from build123d import *

# Parameters (mm, degrees)
BOSS_EXTRUDE1_DEPTH  = 4.7625
M8_CLEARANCE_HOLE1_D = 9
CHAMFER1_SIZE        = 1


with BuildPart() as part:
    # Sketch1 → Boss-Extrude1 (new, symmetric)
    with BuildSketch(Plane.XY):
        Polygon((-17.5, -157.849025767), (5.340097423, -157.849025767), (157.849025767, -5.340097423), (157.849025767, 17.5), (39.267766953, 17.5), (-17.5, -39.267766953), align=None)
    extrude(amount=BOSS_EXTRUDE1_DEPTH, both=True)

    # M8 Clearance Hole1 (through all)
    with Locations(Plane.XY.offset(4.7625)):
        with Locations((0, -92.478445072), (144.956890143, 0), (92.478445072, 0), (0, -40), (0, -144.956890143), (40, 0)):
            Hole(M8_CLEARANCE_HOLE1_D / 2)

    # Chamfer1
    chamfer1_edges = [part.edges().sort_by_distance(p)[0] for p in [
        (157.849025767, 17.5, 0),
        (157.849025767, -5.340097423, 0),
        (5.340097423, -157.849025767, 0),
        (-17.5, -157.849025767, 0),
        (-17.5, -39.267766953, 0),
        (39.267766953, 17.5, 0),
    ]]
    chamfer(chamfer1_edges, length=CHAMFER1_SIZE)


solid = part.part
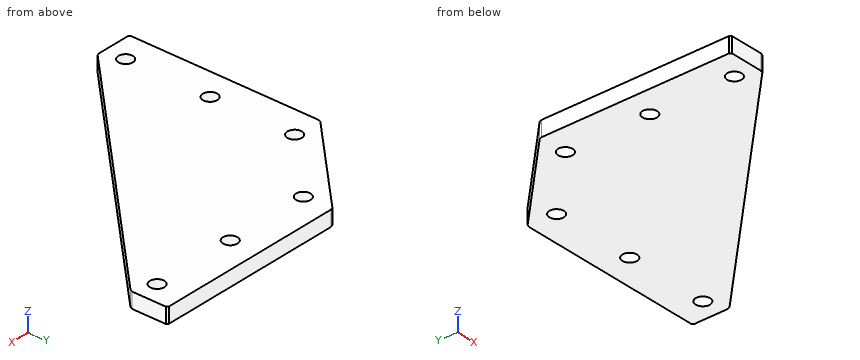
Geometry: final body of the model. Coordinates: model frame, mm. Give positions to 0.01 mm unless a question says otherwise; leave off trailing zeros. Write each loop counter-clockwise with the first axis right and the second up, starting at its lowest first coordinate (ties: lowest second). Pieces come first, ordered by that corner, then holes. Notation, with made-up numbers: (27.25, 56.5) - (65.25, 56.5) arc R13 cw to (65.25, 67.5) - close; hole circle Ø9 at (64.5, 24.5). An arc over 180 degrees is marked (long way). Return JSON: item names as keys, results as strings. Group by question number.
1) Section B-B on y = 0. Return the cut outline in (x, z).
2) First-contact query: P1, Ø7, axis at x = 0, y = -40, coming from the -Z side; P2, Ø10.5, axis at x = 144.96, y = 0, coming from the +Z side; P3, Ø1, axis at y = -94.5, z = 0, coming from the +X side. Flat tips, straight axial feed; report the tip coordinate or a pass-through.
3) Section A-A on z = -1.5. Return the cut outline in (x, y).
4) Line query: line 1 (Y direction, x = 0, z = 1.5); line 2 (Y direction, x = 142.5, z = 0.5); line 3 (Y direction, x = 149, z = -3.25). Output: solid intervals per line, ascending.
5) Section D-D on y = -132.5. Return the cut outline in (x, z), plus the area to 3 significant figures.
6) Section C-C on x = 0. Return the cut outline in (y, z).
Filled in:
{
 "1": {"outline": "(21.77, -4.76) - (35.5, -4.76) - (35.5, 4.76) - (21.77, 4.76) - close; (44.5, -4.76) - (87.98, -4.76) - (87.98, 4.76) - (44.5, 4.76) - close; (96.98, -4.76) - (140.46, -4.76) - (140.46, 4.76) - (96.98, 4.76) - close; (149.46, -4.76) - (157.85, -4.76) - (157.85, 4.76) - (149.46, 4.76) - close"},
 "2": {"P1": "passes through", "P2": "stops at z = 4.76", "P3": "stops at x = 69.19"},
 "3": {"outline": "(-17.5, -156.85) - (-16.5, -157.85) - (4.34, -157.85) - (6.05, -157.14) - (157.14, -6.05) - (157.85, -4.34) - (157.85, 16.5) - (156.85, 17.5) - (40.27, 17.5) - (38.56, 16.79) - (-16.79, -38.56) - (-17.5, -40.27) - close; hole circle Ø9 at (0, -144.96); hole circle Ø9 at (0, -92.48); hole circle Ø9 at (0, -40); hole circle Ø9 at (40, 0); hole circle Ø9 at (92.48, 0); hole circle Ø9 at (144.96, 0)"},
 "4": {"line 1": "y = -157.85 to -149.46, -140.46 to -96.98, -87.98 to -44.5, -35.5 to -21.77", "line 2": "y = -20.69 to -3.77, 3.77 to 17.5", "line 3": "y = -14.19 to -1.98, 1.98 to 17.5"},
 "5": {"outline": "(-17.5, -4.76) - (30.69, -4.76) - (30.69, 4.76) - (-17.5, 4.76) - close", "area": "459 mm^2"},
 "6": {"outline": "(-157.85, -4.76) - (-149.46, -4.76) - (-149.46, 4.76) - (-157.85, 4.76) - close; (-140.46, -4.76) - (-96.98, -4.76) - (-96.98, 4.76) - (-140.46, 4.76) - close; (-87.98, -4.76) - (-44.5, -4.76) - (-44.5, 4.76) - (-87.98, 4.76) - close; (-35.5, -4.76) - (-21.77, -4.76) - (-21.77, 4.76) - (-35.5, 4.76) - close"}
}
